from build123d import *

# Parameters (mm, degrees)
BOSS_EXTRUDE1_DEPTH = 8
SKETCH3_W           = 22.2
SKETCH3_H           = 11.5
CUT_EXTRUDE1_DEPTH  = 8
SKETCH4_R           = 2.5
CUT_EXTRUDE2_DEPTH  = 20
SKETCH6_W           = 5.014738262
SKETCH6_H           = 11.5
CUT_EXTRUDE3_DEPTH  = 1


with BuildPart() as part:
    # Sketch1 → Boss-Extrude1 (new body)
    with BuildSketch(Plane.XY):
        with BuildLine():
            Line((-35, 20), (-35, 10))
            Line((-35, 10), (-55.909806165, 7.44461233))
            ThreePointArc((-55.909806165, 7.44461233), (-50.028760026, 5.615761134), (-47.5, 0))
            ThreePointArc((-47.5, 0), (-50.028760026, -5.615761134), (-55.909806165, -7.44461233))
            Line((-55.909806165, -7.44461233), (-35, -10))
            Line((-35, -10), (-35, -25))
            Line((-35, -25), (35, -25))
            Line((35, -25), (35, 20))
            ThreePointArc((35, 20), (33.535533906, 23.535533906), (30, 25))
            Line((30, 25), (-30, 25))
            ThreePointArc((-30, 25), (-33.535533906, 23.535533906), (-35, 20))
        make_face()
        with BuildLine():
            ThreePointArc((-47.5, 0), (-50.028760026, 5.615761134), (-55.909806165, 7.44461233))
            ThreePointArc((-55.909806165, 7.44461233), (-62.5, 0), (-55.909806165, -7.44461233))
            ThreePointArc((-55.909806165, -7.44461233), (-50.028760026, -5.615761134), (-47.5, 0))
        make_face()
    extrude(amount=BOSS_EXTRUDE1_DEPTH)

    # Sketch3 → Cut-Extrude1 (cut)
    with BuildSketch(Plane.XY.offset(8)):
        with Locations((8.9, 0)):
            Rectangle(SKETCH3_W, SKETCH3_H)
    extrude(amount=-CUT_EXTRUDE1_DEPTH, mode=Mode.SUBTRACT)

    # Sketch4 → Cut-Extrude2 (cut)
    with BuildSketch(Plane.XY.offset(8)):
        with Locations((-52.5, 0)):
            Circle(SKETCH4_R)
    extrude(amount=-CUT_EXTRUDE2_DEPTH, mode=Mode.SUBTRACT)

    # Sketch6 → Cut-Extrude3 (cut)
    with BuildSketch(Plane.XY.offset(8)):
        with Locations((-4.707369131, 0)):
            Rectangle(SKETCH6_W, SKETCH6_H)
        with Locations((22.507369131, 0)):
            Rectangle(SKETCH6_W, SKETCH6_H)
    extrude(amount=-CUT_EXTRUDE3_DEPTH, mode=Mode.SUBTRACT)


solid = part.part
The listing builds one solid part. Answer for the finished solid, in the listing's coordinates (mm). A direction names the side the tool comes from. Coordinates: 2 decimals unless noted, no trailing zeros. Loops run counter-clockwise (first coordinate to the right, second up) from the corner with the lowest first, then second, coordinate; pieces in that order, holes last. Notation, with made-up numbers: M 4.25,10 L 50.25,10 A29 cw 50.25,37 Z; hole C -37.75,23 d4. An arc over 180 degrees is marked long. Answer in a Markdown table with one row per item.
1) Find section C-C (x = -54). Determine the outline of the cut face in (y, z).
Answers below:
| item | result |
|---|---|
| outline | M -7.68,0 L -2,0 L -2,8 L -7.68,8 Z; M 2,0 L 7.68,0 L 7.68,8 L 2,8 Z |
2) Which of the six approach directions +Z, -Z, +X, -X, +Y, -Y give full straight-line access (tool end or side, diameter ignored) to faces 1 (the flat face through (-35, -17, 4)), 2 (the flat face through (-5, 0, 7)), 3 (the flat face through (20, 0, 4)), 4 (the cylindrical face through (-62.5, 0.15, 3.94)), 5 (the cylindrical face through (-33, 24, 4))?
Answers below:
| item | result |
|---|---|
| face 1 | +Z, -Z, -X, -Y |
| face 2 | +Z |
| face 3 | +Z, -Z |
| face 4 | +Z, -Z, -X |
| face 5 | +Z, -Z, -X, +Y |
3) Find the intervals of material crossed by probe 1 along Y at (x, z) = (-52, 1.75); probe 2 along Y at (x, z) = (-52.5, 1.75); probe 3 along X at (y, z) = (-12.5, 7.75), in increasing order.
Answers below:
| item | result |
|---|---|
| probe 1 | -7.92 to -2.45, 2.45 to 7.92 |
| probe 2 | -7.86 to -2.5, 2.5 to 7.86 |
| probe 3 | -35 to 35 |
4) Find section A-A (z = 5). Determine the outline of the cut face in (x, y).
Answers below:
| item | result |
|---|---|
| outline | M -55.91,-7.44 L -35,-10 L -35,-25 L 35,-25 L 35,20 A5 ccw 30,25 L -30,25 A5 ccw -35,20 L -35,10 L -55.91,7.44 A7.5 ccw Z; hole C -52.5,0 d5; hole M -2.2,-5.75 L 20,-5.75 L 20,5.75 L -2.2,5.75 Z |
5) Given pin 1 (0.8 mm diameter, centred on y = -1.5, z = 7.5, fed in from -X); pin 2 (2.5 mm diameter, centred on x = 22.5, y = 1.5, fed in from +Z); pin 3 (1.5 mm diameter, centred on y = -11, z = 3, fed in from -X), each flat-ended and moving along its own axis, determine where each tip first touches the part or whether it passes through.
Answers below:
| item | result |
|---|---|
| pin 1 | x = -62.42 |
| pin 2 | z = 7 |
| pin 3 | x = -35 |
6) Find section D-D (x = 22). Determine the outline of the cut face in (y, z), then the cut area to 4 significant figures.
Answers below:
| item | result |
|---|---|
| outline | M -25,0 L 25,0 L 25,8 L 5.75,8 L 5.75,7 L -5.75,7 L -5.75,8 L -25,8 Z |
| area | 388.5 mm^2 |
7) Find section B-B (y = 0). Determine the outline of the cut face in (x, z).
Answers below:
| item | result |
|---|---|
| outline | M -62.5,0 L -55,0 L -55,8 L -62.5,8 Z; M -50,0 L -2.2,0 L -2.2,7 L -7.21,7 L -7.21,8 L -50,8 Z; M 20,0 L 35,0 L 35,8 L 25.01,8 L 25.01,7 L 20,7 Z |
8) Determine the mould class of faces 6 (the flat face through (22, 0, 7)), 7 (the flat face through (-35, 15, 4)), 8 (the flat face through (9, 5.75, 4)), 9 (the cylindrical face through (34, 23, 4)) for opening direction X: released by +X, released by -X, zero draft, split by the parting line, or undercut.
Answers below:
| item | result |
|---|---|
| face 6 | undercut |
| face 7 | released by -X |
| face 8 | undercut |
| face 9 | released by +X |
